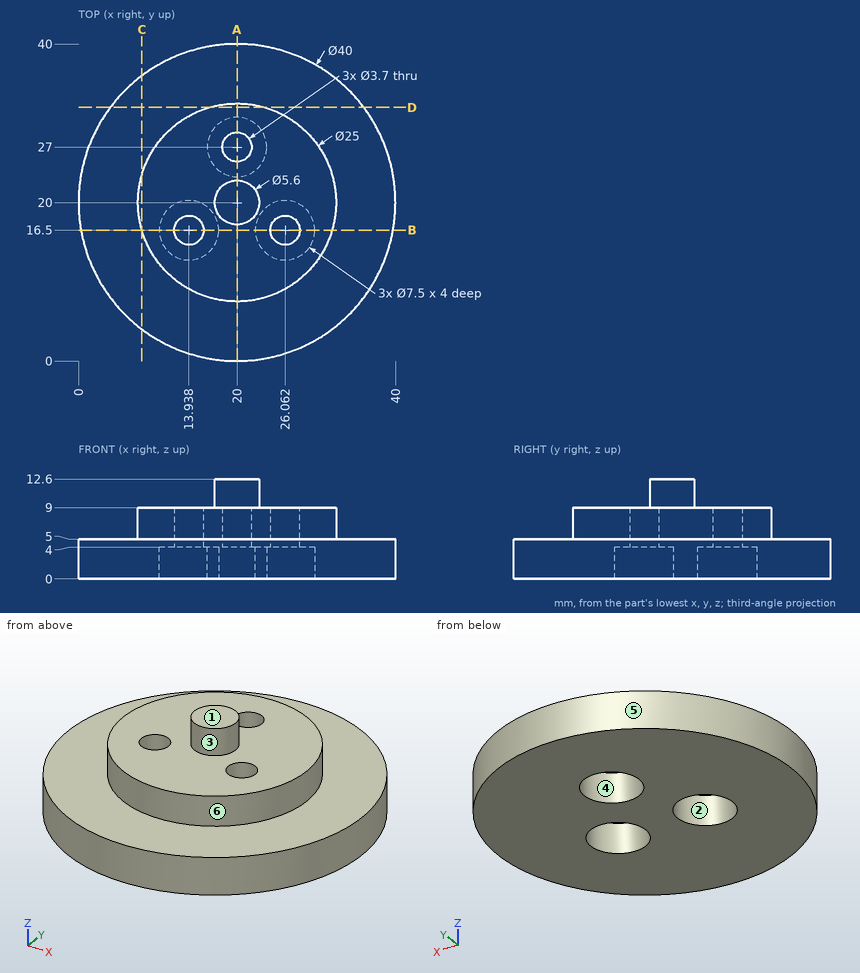
Answer from the drawing. Dimensions are ordinates in mm from the lowest x, y and z of the part. A direction names the side the tool comes from. Round coordinates to 2 decimals unless told otherwise and drop trailing zeros. Write each loop counter-clockwise with the first axis right and the second up, starting at its lowest first coordinate (ties: lowest second). Pieces come first, ordered by that corner, then holes. Notation, with made-up numbers: (50.5, 15) - (98.5, 15) arc R17 cw to (98.5, 48) - close; hole circle Ø9 at (18.25, -29). An arc over 180 degrees is marked (long way). Use a Markdown table: item, result.
(1) Straight lines are drawn through the part: line 1 along Y through (x, z) = (20, 2.4); line 2 along Y through (x, z) = (20, 7.05); line 3 along X through (y, z) = (16.5, 6.85). For each, find the intervals that lie inside material, in ascending order. Write a range as [from, to].
Reported:
| item | result |
|---|---|
| line 1 | [0, 23.25], [30.75, 40] |
| line 2 | [7.5, 25.15], [28.85, 32.5] |
| line 3 | [8, 12.09], [15.79, 24.21], [27.91, 32] |
(2) The part is cut by section B-B (y = 16.5). Write down the section's boundary in (x, z), then the cut area to 3 significant figures.
Reported:
| item | result |
|---|---|
| outline | (0.31, 0) - (10.19, 0) - (10.19, 4) - (12.09, 4) - (12.09, 9) - (8, 9) - (8, 5) - (0.31, 5) - close; (15.79, 4) - (17.69, 4) - (17.69, 0) - (22.31, 0) - (22.31, 4) - (24.21, 4) - (24.21, 9) - (15.79, 9) - close; (27.91, 4) - (29.81, 4) - (29.81, 0) - (39.69, 0) - (39.69, 5) - (32, 5) - (32, 9) - (27.91, 9) - close |
| area | 196 mm2 |
(3) The mould has two halves that part along Y. Classify the marked faces 1, 2 and 3: released by +Y, released by -Y, zero draft, split by the parting line, or undercut.
Reported:
| item | result |
|---|---|
| face 1 | zero draft |
| face 2 | undercut |
| face 3 | split by the parting line |
(4) The part is cut by section C-C (x = 8). Write down the section's boundary in (y, z), then the cut area to 3 significant figures.
Reported:
| item | result |
|---|---|
| outline | (4, 0) - (36, 0) - (36, 5) - (23.5, 5) - (23.5, 9) - (16.5, 9) - (16.5, 5) - (4, 5) - close |
| area | 188 mm2 |
(5) The part is cut by section A-A (x = 20). Write down the section's boundary in (y, z).
Reported:
| item | result |
|---|---|
| outline | (0, 0) - (23.25, 0) - (23.25, 4) - (25.15, 4) - (25.15, 9) - (22.8, 9) - (22.8, 12.6) - (17.2, 12.6) - (17.2, 9) - (7.5, 9) - (7.5, 5) - (0, 5) - close; (28.85, 4) - (30.75, 4) - (30.75, 0) - (40, 0) - (40, 5) - (32.5, 5) - (32.5, 9) - (28.85, 9) - close |
(6) Each of these flat-tipped pins is pushed along its axis until it touches: pin 1 Ø6 at (x, y) = (13.94, 16.5) entering from +Z; pin 2 Ø8 at (x, y) = (27.5, 17) entering from -Z; pin 3 Ø6 at (x, y) = (26.06, 16.5) entering from -Z; pin 4 Ø5 at (x, y) = (5, 28.5) entering from +Z. Where does it stop, or does it pass through?
Reported:
| item | result |
|---|---|
| pin 1 | z = 9 |
| pin 2 | z = 0 |
| pin 3 | z = 4 |
| pin 4 | z = 5 |
(7) Which of the six approach directions +Z, -Z, +X, -X, +Y, -Y give full straight-line access (tool end or side, diameter ignored) to the marked faces 4, 5 and 6?
Reported:
| item | result |
|---|---|
| face 4 | -Z |
| face 5 | +Z, -Z |
| face 6 | +Z |
